Source: CAD feature listing. Evaluate the final solid. Frame: model axes, mm. Give positions to 0.01 mm unless a question says otherwise; leave off trailing zeros. Write each loop counter-clockwise with the first axis right and the second up, starting at its lowest first coordinate (ties: lowest second). Pieces come first, ordered by that corner, then holes. Notation, with made-up numbers: (37, 55) -> (57, 55) arc R22 cw to (57, 62) -> close; hole circle Ø4 at (30, 35). An arc over 180 degrees is marked (long way). Answer as a JSON object with one key per item and string values. Group by question number.
Item 1: Pull-direction query (Y, two-part tool) for faces 1 (the face through (316, 0, 8)), 2 (the face through (640, 37, 8)), 3 (the face through (505.663, 321.5, 7.888)), 4 (the face through (609.237, 35.935, 7.888)); classes: pulls with the +Y half, pulls with the -Y half, needs draft (parallel to the pull), parting line crosses it, or undercut.
Item 2: First-contact query: pin 1 Ø1.5 at (y, z) = (143.5, 1.5) entering from +X; pin 2 Ø14.5 at (x, y) = (278.48, 125.02) entering from -Z; pin 3 Ø1 at (y, z) = (368, 7) entering from -X; pin 4 Ø4 at (y, z) = (79.5, 7) entering from -X. Flat tips, straight axial feed; report the tip coordinate or a pass-through.
Item 3: Section query B-B on z = 5.75. Give the number of separate pieces and of enclosed holes in the cut face, plus the area to 3 significant figures.
Item 4: Section query D-D on x = 600. Return the cut outline in (y, z), plus the area to 3 significant figures.
Item 5: Section query C-C on x = 302.5. Return the cut outline in (y, z).
Item 6: Ray query, probe 1 along Y at (x, z) = (279, 12.5); probe 2 along X at (y, z) = (123.5, 11.75); probe 3 along Y at (x, z) = (41, 14.25). Return the intervals inside material, ascending. Write a range as from..to.
Item 7: Section query A-A on x = 40. Return the cut outline in (y, z).
from build123d import *

# Parameters (mm, degrees)
SKETCH2_R           = 27.775
SKETCH2_R_2         = 8
SKETCH2_R_3         = 10
BOSS_EXTRUDE1_DEPTH = 16


with BuildPart() as part:
    # Sketch2 → Boss-Extrude1 (new body)
    with BuildSketch(Plane.XY):
        Polygon((0, 0), (640, 0), (640, 75), (367.510391728, 575), (272.510391728, 575), (0, 75), align=None)
        with Locations((318.4763261, 490)):
            Circle(SKETCH2_R, mode=Mode.SUBTRACT)
        with Locations((278.4763261, 450)):
            Circle(SKETCH2_R_2, mode=Mode.SUBTRACT)
        with Locations((358.4763261, 450)):
            Circle(SKETCH2_R_2, mode=Mode.SUBTRACT)
        with Locations((193.4763261, 350)):
            Circle(SKETCH2_R_3, mode=Mode.SUBTRACT)
        with Locations((443.4763261, 350)):
            Circle(SKETCH2_R_3, mode=Mode.SUBTRACT)
        with Locations((278.4763261, 125.024449421)):
            Circle(SKETCH2_R_2, mode=Mode.SUBTRACT)
        with Locations((358.4763261, 125.024449421)):
            Circle(SKETCH2_R_2, mode=Mode.SUBTRACT)
        with Locations((318.4763261, 75)):
            Circle(SKETCH2_R, mode=Mode.SUBTRACT)
        with Locations((40, 39.764905221)):
            Circle(SKETCH2_R_3, mode=Mode.SUBTRACT)
        with Locations((600, 39.764905221)):
            Circle(SKETCH2_R_3, mode=Mode.SUBTRACT)
    extrude(amount=BOSS_EXTRUDE1_DEPTH)


solid = part.part
Worked answers:
{
 "1": {"face 1": "pulls with the -Y half", "face 2": "needs draft", "face 3": "pulls with the +Y half", "face 4": "undercut"},
 "2": {"pin 1": "x = 603.08", "pin 2": "through", "pin 3": "x = 159.42", "pin 4": "x = 1.36"},
 "3": {"separate pieces": "1", "enclosed holes": "10", "area": "225,000 mm^2"},
 "4": {"outline": "(0, 0) -> (29.76, 0) -> (29.76, 16) -> (0, 16) -> close; (49.76, 0) -> (148.4, 0) -> (148.4, 16) -> (49.76, 16) -> close", "area": "2,050 mm^2"},
 "5": {"outline": "(0, 0) -> (52.28, 0) -> (52.28, 16) -> (0, 16) -> close; (97.72, 0) -> (467.28, 0) -> (467.28, 16) -> (97.72, 16) -> close; (512.72, 0) -> (575, 0) -> (575, 16) -> (512.72, 16) -> close"},
 "6": {"probe 1": "0..117.04, 133.01..442.02, 457.98..575", "probe 2": "26.43..270.62, 286.33..350.62, 366.33..613.57", "probe 3": "0..29.82, 49.71..150.23"},
 "7": {"outline": "(0, 0) -> (29.76, 0) -> (29.76, 16) -> (0, 16) -> close; (49.76, 0) -> (148.39, 0) -> (148.39, 16) -> (49.76, 16) -> close"}
}
